Can you work these out from the model? Positions are in its coordinate system, mm. A direction names the side the tool comes from. Give positions to 0.01 mm unless a question says otherwise; leave off trailing zeros. Loops run counter-clockwise (first coordinate to the right, second up) from the corner with the lowest first, then second, coordinate; pieces in that order, holes last. Notation, with made-up numbers: M -28.5,65 L -4.5,65 A6 cw -4.5,69 Z; hole C 80,27.25 d5. An arc over 180 degrees is marked long. One line per item, written item: value. Start each with the question number.
Autodesk Inventor part; units mm, degrees
ref_plane "YZ Plane" through (0, 0, 0) normal (1, 0, 0) x (0, 1, 0)
ref_plane "XZ Plane" through (0, 0, 0) normal (0, 1, 0) x (-1, 0, 0)
ref_plane "XY Plane" through (0, 0, 0) normal (0, 0, 1) x (1, 0, 0)
sketch "Sketch1" plane through (0, 0, 0) normal (0, 0, 1) x (1, 0, 0)
  line L0 (-50, -57.5) -> (50, -57.5)
  line L1 (50, -57.5) -> (50, 57.5)
  line L2 (50, 57.5) -> (-50, 57.5)
  line L3 (-50, 57.5) -> (-50, -57.5)
  line L4 (-50, -57.5) -> (50, 57.5) construction
  line L5 (50, -57.5) -> (-50, 57.5) construction
  point P0 (0, 0)
  dimension "d0" = 100
  dimension "d1" = 115
extrude "Extrusion1" add sketch "Sketch1" along normal blind 70
sketch "Sketch2" plane through (50, -57.5, 0) normal (1, 0, 0) x (0, 0, -1)
  line L0 (0, 0) -> (0, 115)
  line L1 (0, 115) -> (-5, 115)
  line L2 (-5, 115) -> (-5, 35)
  line L3 (-5, 35) -> (0, 35)
  line L4 (0, 35) -> (0, 115)
  point P0 (0, 57.5)
  point P1 (0, 35)
  dimension "d4" = 5
  dimension "d5" = 80
extrude "Extrusion2" add sketch "Sketch2" along normal blind 30
mirror "Mirror1" about plane through (0, 0, 0) normal (1, 0, 0) of "Extrusion2"
sketch "Sketch3" plane through (0, 0, 70) normal (0, 0, 1) x (1, 0, 0)
  line L0 (-22.5, 37.5) -> (22.5, 37.5)
  line L1 (22.5, 37.5) -> (22.5, -7.5)
  line L2 (22.5, -7.5) -> (-22.5, -7.5)
  line L3 (-22.5, -7.5) -> (-22.5, 37.5)
  line L4 (0, 50) -> (0, -57.5) construction
  line L5 (-50, -57.5) -> (50, -57.5) construction
  line L6 (50, 57.5) -> (-50, 57.5)
  point P0 (0, 0)
  point P1 (22.5, 15)
  dimension "d8" = 45
  dimension "d9" = 45
  dimension "d10" = 20
extrude "Extrusion3" cut sketch "Sketch3" against normal through all
sketch "Sketch4" plane through (-50, -57.5, 70) normal (-1, 0, 0) x (0, 0, 1)
  circle A0 centre (-30, 30) radius 28
  line L0 (0, 115) -> (0, 0)
  line L1 (-70, 0) -> (0, 0)
  point P0 (-70, 57.5)
  dimension "d13" = 56
  dimension "d14" = 30
  dimension "d15" = 30
extrude "Extrusion4" cut sketch "Sketch4" against normal blind 80
sketch "Sketch5" plane through (0, 0, 70) normal (0, 0, 1) x (1, 0, 0)
  line L0 (-20, -2.5) -> (20, -2.5)
  line L1 (20, -2.5) -> (20, 37.5)
  line L2 (20, 37.5) -> (10, 37.5)
  line L3 (10, 37.5) -> (10, 29.5)
  line L4 (10, 29.5) -> (13.2139, 25.6698)
  line L5 (13.2139, 25.6698) -> (-13.2139, 25.6698)
  line L6 (-13.2139, 25.6698) -> (-10, 29.5)
  line L7 (-10, 29.5) -> (-10, 37.5)
  line L8 (-10, 37.5) -> (-20, 37.5)
  line L9 (-20, 37.5) -> (-20, -2.5)
  line L10 (10, 37.5) -> (-10, 37.5)
  line L11 (-22.5, 37.5) -> (22.5, 37.5)
  point P0 (0, 0)
extrude "Extrusion5" add sketch "Sketch5" against normal up to surface (70 mm away) contours L10 L3 L4 L5 L6 L7
fillet "Fillet1" radius 2 11 edges at (50, 0, 70) (0, -57.5, 70) (-50, 0, 70) (0, 57.5, 70) (50, -57.5, 35) (0, -57.5, 0) (50, -40, 0) (-50, -57.5, 35) (50, 57.5, 37.5) (-50, 57.5, 37.5) (-50, -40, 0)
properties part number "Motor_case" material "Iron, Ductile"
Q1. If we mould it in two halves opening along X, with no side actions, what happens to faces 1 (the face through (0, -7.5, 65)), 2 (the face through (-16, 37.5, 35)), 3 (the face through (80, 18, 3)), 4 (the face through (64, -22.5, 3))? For each: released by +X, released by -X, zero draft, split by the parting line, or undercut.
Q2. If we section it at D-D, the plane y = 42: Write out the boundary of the cut face in (x, z), plus the area to 3 significant figures.
Q3. I need wall thicknesses on line 1 along X through (y, z) = (35, 24.5); line 2 along Y through (x, z) = (-33, 40); line 3 along Y through (x, z) = (-1.5, 40). Which ranges of each line are inside material? Lowest first, please.
Q4. Which directions (+Z, -Z, +X, -X, +Y, -Y) give clear straight access to the entire face, cutting with the end or side of a thin tool? Please do faces 5 (the face through (0, -7.5, 10)), 6 (the face through (1, -11, 0)), 7 (the face through (-10.56, -54.834, 33.93)).
Q5. If we section it at A-A, the plane y = 22.5: Write out the boundary of the cut face in (x, z).
Q6. If we section it at B-B, the plane x = -40.5: Write out the boundary of the cut face in (y, z), plus the area to 3 significant figures.
Q7. For P1, Ø3, axis at y = -35, z = 48, coming from the +X side; P2, Ø4, axis at y = -15, z = 43, coming from the -X side; P3, Ø5.5, axis at x = -71, z = 3.5, coming from the -Y side, each with a flat end and sliding along its axis, tell me the tip position at first contact or that it passes through.
Response:
1. face 1: undercut
1. face 2: undercut
1. face 3: released by +X
1. face 4: zero draft
2. outline: M -80,0 L 80,0 L 80,5 L 50,5 L 50,68 A2 ccw 48,70 L -48,70 A2 ccw -50,68 L -50,5 L -80,5 Z
2. area: 7,300 mm^2
3. line 1: -50 to -22.5, -10 to 10, 22.5 to 50
3. line 2: -57.5 to -55.5, 0.5 to 57.5
3. line 3: -57.5 to -55.5, 25.67 to 57.5
4. face 5: +Z, -Z
4. face 6: -Z, +X, -X, +Y, -Y
4. face 7: -X
5. outline: M -80,0 L -22.5,0 L -22.5,70 L -48,70 A2 ccw -50,68 L -50,5 L -80,5 Z; M 22.5,0 L 80,0 L 80,5 L 50,5 L 50,68 A2 ccw 48,70 L 22.5,70 Z
6. outline: M -57.5,2 A2 ccw -55.5,0 L 57.5,0 L 57.5,68 A2 ccw 55.5,70 L -55.5,70 A2 ccw -57.5,68 Z; hole C -27.5,40 d56
6. area: 5,580 mm^2
7. P1: x = 50
7. P2: x = 30
7. P3: y = -22.5
